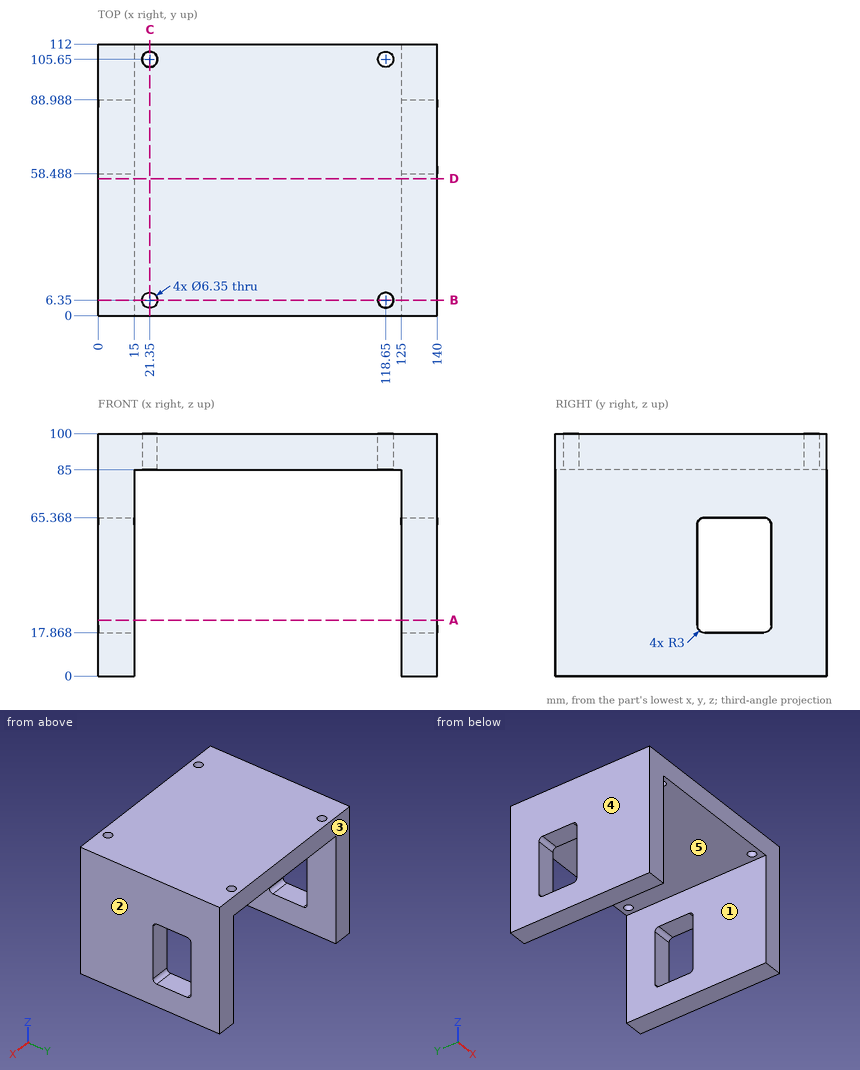
Here's the drawing with two shaded views (mm, measured from the low corner). I have some questions. A direction names the side the tool comes from. Give positions to 0.01 mm unless a question says otherwise; leave off trailing zeros. Loops run counter-clockwise (first coordinate to the right, second up) from the corner with the lowest first, then second, coordinate; pieces in that order, holes last. Notation, with made-up numbers: M 84,44.25 L 132,44.25 A24 ccw 132,71.25 Z; hole C -22,58.5 d2. An arc over 180 degrees is marked long. One line per item, written item: value.
(1) Suppose I cut it at A-A on z = 23. List the corners of the cut face in (x, y) for me.
Returned:
outline: M 0,0 L 15,0 L 15,58.49 L 0,58.49 Z; M 0,88.99 L 15,88.99 L 15,112 L 0,112 Z; M 125,0 L 140,0 L 140,58.49 L 125,58.49 Z; M 125,88.99 L 140,88.99 L 140,112 L 125,112 Z
(2) Which directions (+Z, -Z, +X, -X, +Y, -Y) give clear straight access to the entire face, cutting with the end or side of a thin tool? Please do the marked faces 1 and 2.
Returned:
face 1: -Z, +Y, -Y
face 2: +Z, -Z, +X, +Y, -Y
(3) I need wall thicknesses on line 1 (X direction, y = 105.65, z = 91.25) (1 decimal); line 2 (Y direction, x = 21.35, z = 91) (1 decimal); line 3 (X direction, y = 60.5, z = 68). Which ranges of each line are inside material? Lowest first, please.
Returned:
line 1: 0 to 18.2, 24.5 to 115.5, 121.8 to 140
line 2: 0 to 3.2, 9.5 to 102.5, 108.8 to 112
line 3: 0 to 15, 125 to 140
(4) Suppose I cut it at C-C on x = 21.35. List the corners of the cut face in (y, z) for me (1 decimal).
Returned:
outline: M 0,85 L 3.2,85 L 3.2,100 L 0,100 Z; M 9.5,85 L 102.5,85 L 102.5,100 L 9.5,100 Z; M 108.8,85 L 112,85 L 112,100 L 108.8,100 Z
(5) Suppose I cut it at D-D on y = 56.5. List the corners of the cut face in (x, z) for me, plus the area to 3 significant figures.
Returned:
outline: M 0,0 L 15,0 L 15,85 L 125,85 L 125,0 L 140,0 L 140,100 L 0,100 Z
area: 4,650 mm^2
(6) Will these pins go through, and if not, where does the flat tip stop? pin 1 (10 mm diameter, centred on x = 21.35, y = 105.65, fed in from -Z); pin 2 (5 mm diameter, centred on x = 21.35, y = 6.35, fed in from +Z).
Returned:
pin 1: z = 85
pin 2: through
(7) We'd pull the mould along X, two halves only. Please class the marked faces 3, 4 and 5: released by +X, released by -X, zero draft, split by the parting line, or undercut.
Returned:
face 3: zero draft
face 4: released by -X
face 5: undercut
(8) Suppose I cut it at B-B on y = 6.35. List the corners of the cut face in (x, z) for me (1 decimal).
Returned:
outline: M 0,0 L 15,0 L 15,85 L 18.2,85 L 18.2,100 L 0,100 Z; M 24.5,85 L 115.5,85 L 115.5,100 L 24.5,100 Z; M 121.8,85 L 125,85 L 125,0 L 140,0 L 140,100 L 121.8,100 Z
